Here's how the part is built. I have some questions about the finished solid (model axes, mm). Give positions to 0.01 mm unless a question says otherwise; leave off trailing zeros. Write each loop counter-clockwise with the first axis right and the second up, starting at its lowest first coordinate (ties: lowest second). Pieces come first, ordered by that corner, then holes. Notation, with made-up numbers: (19, 22) -> (42, 22) arc R21 cw to (42, 30) -> close; hole circle Ø5 at (69.25, 40). An arc over 180 degrees is marked (long way). Return JSON: item names as keys, results as strings.
from build123d import *

# Parameters (mm, degrees)
F0_W        = 50.8
F0_H        = 2.794
F1_DEPTH    = 8.89
F2_T1_DEPTH = 66.5602855304
F4_DEPTH    = 25.4


# Not quite as in the source:
# - a fillet or chamfer that OpenCascade refuses, or shapes differently, is made with other operations: its cross-section is extruded or revolved along the edge and cut away or added


with BuildPart() as f1:
    # F0 (on Top) → F1 (new body)
    with BuildSketch(Plane.XY):
        with Locations((0, 1.397)):
            Rectangle(F0_W, F0_H)
    extrude(amount=F1_DEPTH)

    # F2: fillet of radius 3.175 on 1 edges, made by hand

    # F2_s2 → F2_t1 (cut)
    with BuildSketch(Plane.YZ.offset(-33.2801427652)):
        with BuildLine():
            ThreePointArc((2.794, 5.7379428939), (1.9949524406, 7.8439996358), (0, 8.89))
            Line((0, 8.89), (2.794, 8.89))
            Line((2.794, 8.89), (2.794, 5.7379428939))
        make_face()
    extrude(amount=F2_T1_DEPTH, mode=Mode.SUBTRACT)

    # F3 (on face) → F4 (cut)
    with BuildSketch(Plane.XZ):
        with BuildLine():
            ThreePointArc((-22.0345, 8.89), (-21.59, 8.4455), (-21.1455, 8.89))
            Line((-21.1455, 8.89), (-22.0345, 8.89))
        make_face()
        with BuildLine():
            Line((-12.6238, 8.89), (-13.2842, 8.89))
            ThreePointArc((-13.2842, 8.89), (-12.954, 8.5598), (-12.6238, 8.89))
        make_face()
        with BuildLine():
            Line((13.3223, 8.89), (12.5857, 8.89))
            ThreePointArc((12.5857, 8.89), (12.954, 8.5217), (13.3223, 8.89))
        make_face()
        with BuildLine():
            ThreePointArc((21.2852, 8.89), (21.59, 8.5852), (21.8948, 8.89))
            Line((21.8948, 8.89), (21.2852, 8.89))
        make_face()
        with BuildLine():
            Line((-4.0513, 8.89), (-4.5847, 8.89))
            ThreePointArc((-4.5847, 8.89), (-4.318, 8.6233), (-4.0513, 8.89))
        make_face()
        with BuildLine():
            Line((4.7625, 8.89), (3.8735, 8.89))
            ThreePointArc((3.8735, 8.89), (4.318, 8.4455), (4.7625, 8.89))
        make_face()
    extrude(amount=-F4_DEPTH, mode=Mode.SUBTRACT)


solid = f1.part
1. If we mould it in two halves opening along X, with no side actions, what happens to faces 1 (the face through (0, 0, 4)), 2 (the face through (4.308, 0.488, 8.446)), 3 (the face through (-25.4, 1, 4))? For each: released by +X, released by -X, zero draft, split by the parting line, or undercut.
Taken from the geometry:
{"face 1": "zero draft", "face 2": "undercut", "face 3": "released by -X"}
2. For pin 1 Ø4 at (x, z) = (-19.5, 6) entering from +Y; pin 2 Ø2 at (x, z) = (-3, 7.5) entering from +Y, each with a flat end and sliding along its axis, tell me the tip position at first contact or that it passes through.
Taken from the geometry:
{"pin 1": "stops at y = 2.79", "pin 2": "stops at y = 2.7"}
3. Suppose I cut it at B-B, the plane z = 7. List the corners of the cut face in (x, y) for me, and give its area (3 significant figures).
Taken from the geometry:
{"outline": "(-25.4, 0) -> (25.4, 0) -> (25.4, 2.53) -> (-25.4, 2.53) -> close", "area": "129 mm²"}
4. If I drill on line 1 (Z direction, x = -14, y = 0.95); line 2 (Z direction, x = -11, y = 1.15); line 3 (Y direction, x = 12.5, z = 7.5), over which ranges is the centre line in solid material (lowest first)? Write a range as [from, to].
Taken from the geometry:
{"line 1": "z = [0, 8.62]", "line 2": "z = [0, 8.52]", "line 3": "y = [0, 2.26]"}
5. Suppose I cut it at C-C, the plane x = -3.5. List the corners of the cut face in (y, z) for me (3 decimals).
Taken from the geometry:
{"outline": "(0, 0) -> (2.794, 0) -> (2.794, 5.738) arc R3.175 ccw to (0, 8.89) -> close"}
